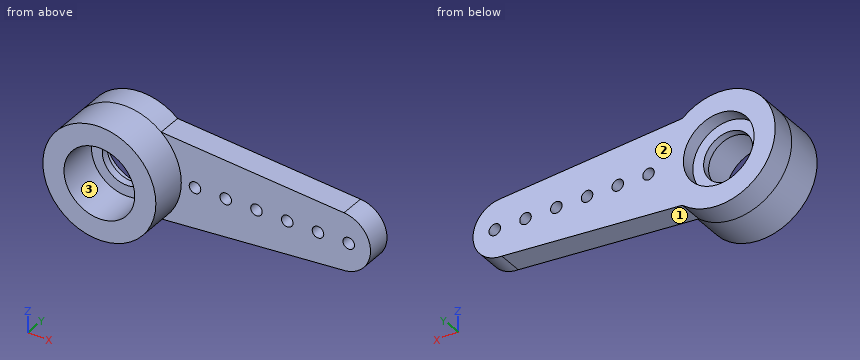
```python
from build123d import *

# Parameters (mm, degrees)
BOSS_EXTRUDE1_DEPTH = 1.62
SKETCH2_R           = 3.675
BOSS_EXTRUDE2_DEPTH = 2.5
SKETCH3_R           = 2.3
SKETCH3_R_2         = 1.6
CUT_EXTRUDE1_DEPTH  = 2.7
SKETCH4_R           = 1.6
CUT_EXTRUDE2_DEPTH  = 4.12
SKETCH5_R           = 2.3
CUT_EXTRUDE3_DEPTH  = 0.93
SKETCH7_R           = 0.375
CUT_EXTRUDE4_DEPTH  = 1.62


with BuildPart() as part:
    # Sketch1 → Boss-Extrude1 (new body)
    with BuildSketch(Plane(origin=(0, 0, 0), x_dir=(1, 0, 0), z_dir=(0, 1, 0))):
        with BuildLine():
            Line((-30.04567513, 12.821055753), (-18.302594635, 11.884771872))
            ThreePointArc((-18.302594635, 11.884771872), (-16.429062652, 10.083953465), (-18.15434761, 8.140641642))
            Line((-18.15434761, 8.140641642), (-30.046970978, 7.197397481))
            ThreePointArc((-30.046970978, 7.197397481), (-36.087594537, 10.010618695), (-30.04567513, 12.821055753))
        make_face()
    extrude(amount=BOSS_EXTRUDE1_DEPTH)

    # Sketch2 → Boss-Extrude2 (add)
    with BuildSketch(Plane.XZ):
        with Locations((-32.412594635, -10.009771872)):
            Circle(SKETCH2_R)
    extrude(amount=BOSS_EXTRUDE2_DEPTH)

    # Sketch3 → Cut-Extrude1 (cut)
    with BuildSketch(Plane.XZ.offset(2.5)):
        with Locations((-32.412594635, -10.009771872)):
            Circle(SKETCH3_R)
        with Locations((-32.412594635, -10.009771872)):
            Circle(SKETCH3_R_2, mode=Mode.SUBTRACT)
    extrude(amount=-CUT_EXTRUDE1_DEPTH, mode=Mode.SUBTRACT)

    # Sketch4 → Cut-Extrude2 (cut)
    with BuildSketch(Plane.XZ.offset(2.5)):
        with Locations((-32.412594635, -10.009771872)):
            Circle(SKETCH4_R)
    extrude(amount=-CUT_EXTRUDE2_DEPTH, mode=Mode.SUBTRACT)

    # Sketch5 → Cut-Extrude3 (cut)
    with BuildSketch(Plane(origin=(0, 1.62, 0), x_dir=(1, 0, 0), z_dir=(0, 1, 0))):
        with Locations((-32.412594635, 10.009771872)):
            Circle(SKETCH5_R)
    extrude(amount=-CUT_EXTRUDE3_DEPTH, mode=Mode.SUBTRACT)

    # Sketch7 → Cut-Extrude4 (cut)
    with BuildSketch(Plane.XZ):
        with Locations((-27.846278089, -10.008997382)):
            Circle(SKETCH7_R)
        with Locations((-25.846278089, -10.008997382)):
            Circle(SKETCH7_R)
        with Locations((-23.846278089, -10.008997382)):
            Circle(SKETCH7_R)
        with Locations((-21.846278089, -10.008997382)):
            Circle(SKETCH7_R)
        with Locations((-19.846278089, -10.008997382)):
            Circle(SKETCH7_R)
        with Locations((-17.846278089, -10.008997382)):
            Circle(SKETCH7_R)
    extrude(amount=-CUT_EXTRUDE4_DEPTH, mode=Mode.SUBTRACT)


solid = part.part
```
CAD build for the part. Positions are in the model's coordinates, mm. Face numbers are marked on the shaded views. Coordinates: 2 decimals unless noted, no trailing zeros. Write each loop counter-clockwise with the first axis right and the second up, starting at its lowest first coordinate (ties: lowest second). Pieces come first, ordered by that corner, then holes. Notation, with made-up numbers: (73, 30) -> (116, 30) arc R28 ccw to (116, 52) -> close; hole circle Ø11 at (6.25, 3.5). An arc over 180 degrees is marked (long way). Return JSON: item names as keys, results as strings. Group by question number.
Q1. Cut at C-C, the plane z = -13. Give the cut face in (x, y), then the cut area to 3 significant figures.
Q2. Cut at D-D, the plane x = -31.5. Give the cut face in (y, z).
Q3. Pull direction X, two halves, no side cores. Call the marked faces 1, 2 and 3: released by +X, released by -X, zero draft, split by the parting line, or undercut.
Q4. Cut at B-B, the plane y = 1. Give the cut face in (x, z) (3 decimals).
Q5. Cut at A-A, the plane x = -21.75. Give the cut face in (y, z).
Q6. Drill centre lines: line 1 (Y direction, x = -28.5, z = -12); line 2 (X direction, y = -0.25, z = -11.25); line 3 (X direction, y = -1, z = -12). Where is each one in solid material? Low to high.
Q7. Flat gauge pins, fed straight in: pin 1 (2 mm diameter, centred on y = -1.5, z = -11, fed in from +X); pin 2 (3.5 mm diameter, centred on x = -32.41, z = -10.01, fed in from -Y); pin 3 (3 mm diameter, centred on x = -21, z = -11.5, fed in from -Y); pin 4 (3 mm diameter, centred on x = -32.41, z = -10.01, fed in from +Y). Where does each tip first touch, or does it go through?
Returned:
{
 "1": {"outline": "(-34.55, -2.5) -> (-30.28, -2.5) -> (-30.28, 1.62) -> (-34.55, 1.62) -> close", "area": "17.6 mm2"},
 "2": {"outline": "(-2.5, -13.57) -> (1.62, -13.57) -> (1.62, -12.12) -> (0.69, -12.12) -> (0.69, -11.32) -> (0.2, -11.32) -> (0.2, -12.12) -> (-2.5, -12.12) -> close; (-2.5, -7.9) -> (0.2, -7.9) -> (0.2, -8.7) -> (0.69, -8.7) -> (0.69, -7.9) -> (1.62, -7.9) -> (1.62, -6.45) -> (-2.5, -6.45) -> close"},
 "3": {"face 1": "released by +X", "face 2": "zero draft", "face 3": "undercut"},
 "4": {"outline": "(-30.047, -7.197) arc R3.675 ccw (long way) to (-30.046, -12.821) -> (-18.303, -11.885) arc R1.875 ccw to (-18.154, -8.141) -> close; hole circle Ø4.6 at (-32.413, -10.01); hole circle Ø0.75 at (-27.846, -10.009); hole circle Ø0.75 at (-25.846, -10.009); hole circle Ø0.75 at (-23.846, -10.009); hole circle Ø0.75 at (-21.846, -10.009); hole circle Ø0.75 at (-19.846, -10.009); hole circle Ø0.75 at (-17.846, -10.009)"},
 "5": {"outline": "(0, -12.16) -> (1.62, -12.16) -> (1.62, -10.37) -> (0, -10.37) -> close; (0, -9.65) -> (1.62, -9.65) -> (1.62, -7.86) -> (0, -7.86) -> close"},
 "6": {"line 1": "y = 0 to 1.62", "line 2": "x = -35.87 to -34.35, -30.48 to -28.95", "line 3": "x = -35.5 to -33.57, -31.26 to -29.32"},
 "7": {"pin 1": "stops at x = -28.74", "pin 2": "stops at y = 0.2", "pin 3": "stops at y = 0", "pin 4": "passes through"}
}
